```python
from build123d import *

# Parameters (mm, degrees)
SKETCH_1_W          = 220
SKETCH_1_H          = 110
EXTRUDE_1_DEPTH     = 3
SKETCH_2_W          = 220
SKETCH_2_H          = 110
CUT_EXTRUDE_1_DEPTH = 10
SKETCH_3_R          = 2.5
SKETCH_3_R_2        = 1.5875
CUT_EXTRUDE_2_DEPTH = 123.752107925
SKETCH_4_R          = 5.5
CUT_EXTRUDE_3_DEPTH = 123.752107925


with BuildPart() as part:
    # Эскиз1 → Бобышка-Вытянуть1 (new body)
    with BuildSketch(Plane(origin=(0, 0, 0), x_dir=(1, 0, 0), z_dir=(0, 1, 0))):
        Rectangle(SKETCH_1_W, SKETCH_1_H)
    extrude(amount=EXTRUDE_1_DEPTH)

    # Эскиз2 → Вырез-Вытянуть1 (cut)
    with BuildSketch(Plane.XZ):
        Rectangle(SKETCH_2_W, SKETCH_2_H)
        with BuildLine():
            ThreePointArc((104, -54.8), (108.101219331, -53.101219331), (109.8, -49))
            Line((109.8, -49), (109.8, 49))
            ThreePointArc((109.8, 49), (108.101219331, 53.101219331), (104, 54.8))
            Line((104, 54.8), (-104, 54.8))
            ThreePointArc((-104, 54.8), (-108.101219331, 53.101219331), (-109.8, 49))
            Line((-109.8, 49), (-109.8, -49))
            ThreePointArc((-109.8, -49), (-108.101219331, -53.101219331), (-104, -54.8))
            Line((-104, -54.8), (104, -54.8))
        make_face(mode=Mode.SUBTRACT)
    extrude(amount=-CUT_EXTRUDE_1_DEPTH, mode=Mode.SUBTRACT)

    # Эскиз3 → Вырез-Вытянуть2 (cut, through all)
    # profile 1 of 5: a face of its own
    with BuildSketch(Plane(origin=(0, 3, 0), x_dir=(1, 0, 0), z_dir=(0, 1, 0))):
        with Locations(Location((-95, 0, 0), (0, 0, 270))):
            Circle(SKETCH_3_R)
        with Locations((-95, 0)):
            Circle(SKETCH_3_R_2, mode=Mode.SUBTRACT)
    # profile 2 of 5: a face of its own
    with BuildSketch(Plane(origin=(0, 3, 0), x_dir=(1, 0, 0), z_dir=(0, 1, 0))):
        with Locations((-95, 0)):
            Circle(SKETCH_3_R_2)
    # profile 3 of 5: a face of its own
    with BuildSketch(Plane(origin=(0, 3, 0), x_dir=(1, 0, 0), z_dir=(0, 1, 0))):
        with Locations(Location((-95, -18, 0), (0, 0, 270))):
            Circle(SKETCH_3_R)
        with Locations((-95, -18)):
            Circle(SKETCH_3_R_2, mode=Mode.SUBTRACT)
    # profile 4 of 5: a face of its own
    with BuildSketch(Plane(origin=(0, 3, 0), x_dir=(1, 0, 0), z_dir=(0, 1, 0))):
        with Locations((-95, -18)):
            Circle(SKETCH_3_R_2)
    # profile 5 of 5: a face of its own
    with BuildSketch(Plane(origin=(0, 3, 0), x_dir=(1, 0, 0), z_dir=(0, 1, 0))):
        with BuildLine():
            ThreePointArc((-101.5, -13), (-97.5, -9), (-101.5, -5))
            Line((-101.5, -5), (-109.8, -5))
            Line((-109.8, -5), (-109.8, -13))
            Line((-109.8, -13), (-101.5, -13))
        make_face()
    extrude(amount=-CUT_EXTRUDE_2_DEPTH, mode=Mode.SUBTRACT)

    # Эскиз4 → Вырез-Вытянуть3 (cut, through all)
    with BuildSketch(Plane(origin=(0, 3, 0), x_dir=(1, 0, 0), z_dir=(0, 1, 0))):
        with Locations(Location((0, 22.5, 0), (0, 0, 270))):
            Circle(SKETCH_4_R)
        with Locations(Location((0, -22.5, 0), (0, 0, 270))):
            Circle(SKETCH_4_R)
    extrude(amount=-CUT_EXTRUDE_3_DEPTH, mode=Mode.SUBTRACT)


solid = part.part
```
Can you work these out from the model? Positions are in its coordinate system, mm. Give positions to 0.01 mm unless a question says otherwise; leave off trailing zeros. Write each loop counter-clockwise with the first axis right and the second up, starting at its lowest first coordinate (ties: lowest second). Pieces come first, ordered by that corner, then holes. Notation, with made-up numbers: (18.5, -39) -> (62.5, -39) arc R11 ccw to (62.5, -34) -> close; hole circle Ø4 at (51, -23.75). An arc over 180 degrees is marked (long way). Write item = value, one per line.
(1) Suppose I cut it at A-A on z = 0. Write out the boundary of the cut face in (x, y).
Worked out:
outline = (-109.8, 0) -> (-97.5, 0) -> (-97.5, 3) -> (-109.8, 3) -> close; (-92.5, 0) -> (109.8, 0) -> (109.8, 3) -> (-92.5, 3) -> close
(2) I'm going to push flat-ended pins straight in: P1, Ø9, axis at x = 0, z = -22.5, coming from the +Y side; P2, Ø8, axis at x = -95, z = 0, coming from the -Y side. Where does each tip first touch, or does it pass through?
Worked out:
P1 = through
P2 = 0
(3) I need wall thicknesses on probe 1 along X at (y, z) = (1.45, 22.5); probe 2 along X at (y, z) = (1.1, 17.5); probe 3 along X at (y, z) = (1.7, 18). Which ranges of each line are inside material? Lowest first, please. Write a range as from..to.
Worked out:
probe_1 = -109.8..-5.5, 5.5..109.8
probe_2 = -109.8..-97.45, -92.55..-2.29, 2.29..109.8
probe_3 = -109.8..-97.5, -92.5..-3.16, 3.16..109.8
(4) Suppose I cut it at B-B on z = -22.5. Write out the boundary of the cut face in (x, y).
Worked out:
outline = (-109.8, 0) -> (-5.5, 0) -> (-5.5, 3) -> (-109.8, 3) -> close; (5.5, 0) -> (109.8, 0) -> (109.8, 3) -> (5.5, 3) -> close
(5) Thinking about a two-plate mould opening in Z: for faces 1 (the face through (108.1, 1.5, 53.1)), 2 (the face through (-2, 3, -1)), 3 (the face through (1.652, 1.521, -17.254)), which applies, released by +Z, released by -Z, zero draft, split by the parting line, or undercut?
Worked out:
face_1 = released by +Z
face_2 = zero draft
face_3 = undercut
(6) Suppose I cut it at C-C on x = 2.5. Write out the boundary of the cut face in (y, z).
Worked out:
outline = (0, -54.8) -> (3, -54.8) -> (3, -27.4) -> (0, -27.4) -> close; (0, -17.6) -> (3, -17.6) -> (3, 17.6) -> (0, 17.6) -> close; (0, 27.4) -> (3, 27.4) -> (3, 54.8) -> (0, 54.8) -> close
